```python
from build123d import *

# Parameters (mm, degrees)
SKETCH1_R           = 5
SKETCH1_R_2         = 1.1
SKETCH1_R_3         = 4
BOSS_EXTRUDE1_DEPTH = 3
SKETCH2_R           = 1.35
SKETCH2_W           = 10
SKETCH2_H           = 3
CUT_EXTRUDE2_DEPTH  = 5
CUT_EXTRUDE3_START  = -3
CUT_EXTRUDE3_DEPTH  = 3


with BuildPart() as part:
    # Sketch1 → Boss-Extrude1 (new body)
    with BuildSketch(Plane.XY):
        with BuildLine():
            ThreePointArc((-11.658277887, -20.5832063), (-39.551034339, -17.233624375), (-27.264419704, -42.497524754))
            add(Edge.make_bspline(
                [(-27.264419704, -42.497524754), (-25.334460253, -42.955768201), (-21.452320642, -43.816124737), (-13.705385842, -45.286858174), (-4.006421964, -46.667533574), (7.638269658, -47.586831656), (19.289241844, -47.768762722), (30.941925955, -47.212824411), (42.591601286, -45.920000504), (52.298162816, -44.228522597), (60.052175742, -42.510146288), (63.940283625, -41.52535362), (65.871739475, -41.00572578)],
                knots=[0.004189422, 0.004189422, 0.004189422, 0.004189422, 0.066427583, 0.128665745, 0.253142067, 0.377618389, 0.502094711, 0.626571033, 0.751047356, 0.875523678, 0.937761839, 1, 1, 1, 1], degree=3))
            add(Edge.make_bspline(
                [(68.935876888, -41.399946265), (67.056778784, -40.529280178), (65.871739475, -41.00572578)],
                knots=[0, 0, 0, 1, 1, 1], degree=2))
            ThreePointArc((68.935876888, -41.399946265), (91.352405248, -26.204284986), (67.957252813, -12.563327983))
            add(Edge.make_bspline(
                [(67.957252813, -12.563327983), (65.455609859, -13.713888582), (60.364787712, -15.882927404), (52.683559955, -18.641296662), (44.896066709, -20.933273776), (37.015370972, -22.752952432), (29.033864031, -24.103049266), (20.950849492, -24.983508442), (14.12359191, -25.325141054), (8.614596461, -25.364124484), (5.82883012, -25.303122311), (4.440642397, -25.254725163)],
                knots=[0.003418543, 0.003418543, 0.003418543, 0.003418543, 0.119867337, 0.236316132, 0.352764926, 0.46921372, 0.585662514, 0.702111309, 0.818560103, 0.8767845, 0.935008897, 0.935008897, 0.935008897, 0.935008897], degree=3))
            add(Edge.make_bspline(
                [(-11.658277887, -20.5832063), (-9.065688302, -25.060046308), (4.440642397, -25.254725163)],
                knots=[0, 0, 0, 1, 1, 1], degree=2))
        make_face()
        with Locations((75.361610976, -26.74696222)):
            Circle(SKETCH1_R, mode=Mode.SUBTRACT)
        with Locations((75.361610976, -18.74696222)):
            Circle(SKETCH1_R_2, mode=Mode.SUBTRACT)
        with Locations((81.018465226, -21.090107971)):
            Circle(SKETCH1_R_2, mode=Mode.SUBTRACT)
        with Locations((83.361610976, -26.74696222)):
            Circle(SKETCH1_R_2, mode=Mode.SUBTRACT)
        with Locations((-26.518107506, -26.514939916)):
            Circle(SKETCH1_R_3, mode=Mode.SUBTRACT)
        with Locations((81.018465226, -32.40381647)):
            Circle(SKETCH1_R_2, mode=Mode.SUBTRACT)
        with Locations((-26.516504294, -18.516504294)):
            Circle(SKETCH1_R_2, mode=Mode.SUBTRACT)
        with Locations((-20.859650045, -20.859650045)):
            Circle(SKETCH1_R_2, mode=Mode.SUBTRACT)
        with Locations((-18.516504294, -26.516504294)):
            Circle(SKETCH1_R_2, mode=Mode.SUBTRACT)
        with Locations((-20.859650045, -32.173358544)):
            Circle(SKETCH1_R_2, mode=Mode.SUBTRACT)
        with Locations((-26.516504294, -34.516504294)):
            Circle(SKETCH1_R_2, mode=Mode.SUBTRACT)
        with Locations((-32.173358544, -32.173358544)):
            Circle(SKETCH1_R_2, mode=Mode.SUBTRACT)
        with Locations((-34.516504294, -26.516504294)):
            Circle(SKETCH1_R_2, mode=Mode.SUBTRACT)
        with Locations((-32.173358544, -20.859650045)):
            Circle(SKETCH1_R_2, mode=Mode.SUBTRACT)
        with Locations((75.361610976, -34.74696222)):
            Circle(SKETCH1_R_2, mode=Mode.SUBTRACT)
        with Locations((69.704756727, -32.40381647)):
            Circle(SKETCH1_R_2, mode=Mode.SUBTRACT)
        with Locations((67.361610976, -26.74696222)):
            Circle(SKETCH1_R_2, mode=Mode.SUBTRACT)
        with Locations((69.704756727, -21.090107971)):
            Circle(SKETCH1_R_2, mode=Mode.SUBTRACT)
    extrude(amount=BOSS_EXTRUDE1_DEPTH)

    # Sketch2 → Cut-Extrude2 (cut)
    with BuildSketch(Plane.XY.offset(3)):
        with Locations((25.361610976, -31.831277184)):
            Circle(SKETCH2_R)
        with Locations((25.361610976, -39.625455239)):
            Circle(SKETCH2_R)
        with Locations((25.361610976, -25.331277184)):
            Rectangle(SKETCH2_W, SKETCH2_H)
        with Locations((25.361610976, -46.125455239)):
            Rectangle(SKETCH2_W, SKETCH2_H)
    extrude(amount=-CUT_EXTRUDE2_DEPTH, mode=Mode.SUBTRACT)

    # Sketch3 → Cut-Extrude3 (cut)
    with BuildSketch(Plane.XY.offset(3).offset(CUT_EXTRUDE3_START)):
        with BuildLine():
            Line((17.361610979, -32.847645213), (17.361610979, -40.364046911))
            ThreePointArc((17.361610979, -40.364046911), (17.283764857, -40.567864243), (17.089867993, -40.667891887))
            add(Edge.make_bspline(
                [(-14.312749434, -38.014569119), (-14.269650418, -38.022037001), (-14.226551001, -38.029489198), (-10.363330527, -38.696055752), (-6.541302391, -39.231722676), (3.882945868, -40.354666967), (10.485495494, -40.696055442), (17.089867993, -40.667891887)],
                knots=[0.247179417, 0.247179417, 0.247179417, 0.247179417, 0.25, 0.25, 0.5, 0.5, 0.932004212, 0.932004212, 0.932004212, 0.932004212], degree=3))
            ThreePointArc((-14.312749434, -38.014569119), (-14.669439204, -37.639304361), (-14.551126107, -37.135267416))
            ThreePointArc((-14.551126107, -37.135267416), (-12.411809014, -34.065591732), (-11.04390733, -30.583001975))
            ThreePointArc((-11.04390733, -30.583001975), (-10.714611633, -30.151374436), (-10.176280778, -30.081104386))
            add(Edge.make_bspline(
                [(4.267556159, -32.252928603), (1.852622916, -32.216188916), (-0.375859274, -32.085089658), (-3.492192372, -31.719262737), (-4.49789731, -31.56771677), (-6.440834889, -31.196104486), (-7.378139349, -30.976217552), (-8.930356181, -30.525801619), (-9.55919338, -30.317521868), (-10.176280778, -30.081104386)],
                knots=[0.002464962, 0.002464962, 0.002464962, 0.002464962, 0.25, 0.25, 0.375, 0.375, 0.5, 0.5, 0.588245737, 0.588245737, 0.588245737, 0.588245737], degree=3))
            add(Edge.make_bspline(
                [(16.700596662, -32.184353658), (15.333410228, -32.248220782), (13.962679354, -32.293390217), (11.198499486, -32.34676917), (9.803462323, -32.354507183), (7.02323328, -32.330858195), (5.642167753, -32.300269863), (4.267556159, -32.252928603)],
                knots=[0.252874617, 0.252874617, 0.252874617, 0.252874617, 0.5, 0.5, 0.75, 0.75, 0.995779377, 0.995779377, 0.995779377, 0.995779377], degree=3))
            ThreePointArc((16.700596662, -32.184353658), (17.168142051, -32.37943169), (17.361610979, -32.847645213))
        make_face()
        with BuildLine():
            Line((33.361610975, -31.278823407), (33.361610975, -38.949732453))
            ThreePointArc((33.361610975, -38.949732453), (33.595821002, -39.524545963), (34.165063011, -39.771989778))
            add(Edge.make_bspline(
                [(34.165063011, -39.771989778), (38.42004494, -39.343698243), (42.676282868, -38.762038611), (49.786416711, -37.534421652), (52.637938271, -36.973469388), (56.916570991, -36.028567717), (58.344097641, -35.696067505), (60.144263746, -35.255068175), (60.515405719, -35.16298747), (60.886425955, -35.069780201)],
                knots=[0.126769028, 0.126769028, 0.126769028, 0.126769028, 0.5, 0.5, 0.75, 0.75, 0.875, 0.875, 0.907463599, 0.907463599, 0.907463599, 0.907463599], degree=3))
            ThreePointArc((60.886425955, -35.069780201), (61.228166777, -34.682653023), (61.186664011, -34.167937798))
            ThreePointArc((61.186664011, -34.167937798), (59.68189337, -29.932312404), (59.414647943, -25.445282536))
            ThreePointArc((59.414647943, -25.445282536), (59.051007293, -24.46828568), (58.067846264, -24.121656525))
            add(Edge.make_bspline(
                [(58.067846264, -24.121656525), (55.872279142, -24.895690317), (53.666529644, -25.614427728), (45.723836534, -27.994487025), (39.921526423, -29.346512462), (34.043951004, -30.334640585)],
                knots=[0.33139413, 0.33139413, 0.33139413, 0.33139413, 0.5, 0.5, 0.934761271, 0.934761271, 0.934761271, 0.934761271], degree=3))
            ThreePointArc((34.043951004, -30.334640585), (33.550050234, -30.69635686), (33.361610975, -31.278823407))
        make_face()
    extrude(amount=CUT_EXTRUDE3_DEPTH, mode=Mode.SUBTRACT)


solid = part.part
```
Here's how the part is built. I have some questions about the finished solid (model axes, mm). A direction names the side the tool comes from. Give positions to 0.01 mm unless a question says otherwise; leave off trailing zeros. Answer as a JSON object with one key per item and string values. Group by question number.
Item 1: Please list where these lines run through material, in increasing order: probe 1 along Y at (x, z) = (15, 1); probe 2 along Y at (x, z) = (74.5, 0.8); probe 3 along Y at (x, z) = (52, 2.3).
Item 2: For P1, Ø1.8, axis at x = -18.52, y = -26.52, coming from the +Z side; P2, Ø1, axis at y = -22, z = 1, coming from the +X side; P3, Ø1.5, axis at y = -25.5, z = 2, coming from the +X side; P4, Ø1.5, axis at x = 23, z = 1, coming from the +Y side, each with a flat end and sliding along its axis, tell me the tip position at first contact or that it passes through.
Item 3: If we mould it in two halves opening along X, with no side actions, what happens to faces 4 (the flat face through (23, -29, 0)), 5 (the cylindrical face through (-12.437, -34.112, 1.479)), 6 (the cylindrical face through (-32.984, -20.116, 1.479))? For each: pulls with the +X half, pulls with the -X half, needs draft (parallel to the pull), parting line crosses it, or undercut.
Item 4: If we section it at A-A on z = 1.85: Give the number of separate pieces and of enclosed holes in the cut face, and give its area (3 significant figures).
Item 5: Which directions (+Z, -Z, +X, -X, +Y, -Y) give clear straight access to the entire face, cutting with the end or side of a thin tool? Please do faces 1 (the flat face through (25, -26.831, 2)), 2 (the flat face through (20.362, -46, 2)), 3 (the cylindrical face through (59.695, -29.994, 1.479)).
Result set:
{
 "1": {"probe 1": "-47.66 to -40.66, -32.25 to -25.25", "probe 2": "-42.72 to -35.43, -34.06 to -31.67, -21.82 to -19.43, -18.06 to -10.77", "probe 3": "-44.22 to -37.08, -26.11 to -18.78"},
 "2": {"P1": "through", "P2": "x = 90.79", "P3": "x = 91.35", "P4": "y = -26.83"},
 "3": {"face 4": "needs draft", "face 5": "undercut", "face 6": "undercut"},
 "4": {"separate pieces": "1", "enclosed holes": "22", "area": "2,610 mm²"},
 "5": {"face 1": "+Z, -Z, +Y", "face 2": "+Z, -Z, -Y", "face 3": "+Z, -Z"}
}
